from build123d import *

# Parameters (mm, degrees)
BOSS_EXTRUDE1_DEPTH = 1.5875
SKETCH2_W           = 43
SKETCH2_H           = 127
BOSS_EXTRUDE2_DEPTH = 1.5875


with BuildPart() as part:
    # Sketch1 → Boss-Extrude1 (new body)
    with BuildSketch(Plane.XY):
        Polygon((-117, 99.5), (-103.5, 116.5), (-103.5, 120), (-146.5, 120), (-146.5, 116.5), (-133, 99.5), (-133, 20.5), (-146.5, 3.5), (-146.5, 0), (-103.5, 0), (-103.5, 3.5), (-117, 20.5), align=None)
        with BuildLine():
            ThreePointArc((-134.15, 112.5), (-132.5, 110.85), (-130.85, 112.5))
            ThreePointArc((-130.85, 112.5), (-132.5, 114.15), (-134.15, 112.5))
        make_face(mode=Mode.SUBTRACT)
        with BuildLine():
            ThreePointArc((-119.15, 112.5), (-117.5, 110.85), (-115.85, 112.5))
            ThreePointArc((-115.85, 112.5), (-117.5, 114.15), (-119.15, 112.5))
        make_face(mode=Mode.SUBTRACT)
        with BuildLine():
            ThreePointArc((-115.85, 7.5), (-117.5, 9.15), (-119.15, 7.5))
            ThreePointArc((-119.15, 7.5), (-117.5, 5.85), (-115.85, 7.5))
        make_face(mode=Mode.SUBTRACT)
        with BuildLine():
            ThreePointArc((-134.15, 7.5), (-132.5, 5.85), (-130.85, 7.5))
            ThreePointArc((-130.85, 7.5), (-132.5, 9.15), (-134.15, 7.5))
        make_face(mode=Mode.SUBTRACT)
    extrude(amount=BOSS_EXTRUDE1_DEPTH)

    # Sketch2 → Boss-Extrude2 (add)
    with BuildSketch(Plane(origin=(0, 120, 0), x_dir=(1, 0, 0), z_dir=(0, 1, 0))):
        with Locations((-125, 61.9125)):
            Rectangle(SKETCH2_W, SKETCH2_H)
    extrude(amount=BOSS_EXTRUDE2_DEPTH)


solid = part.part
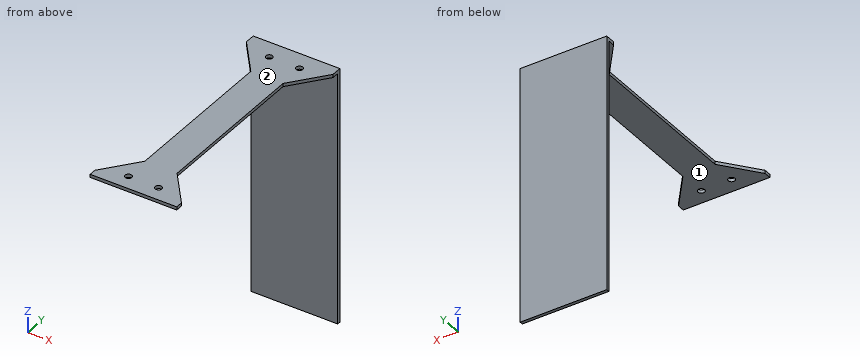
Input: part model. Units: mm. Frame: model coordinates. Face numbers are marked on the shaded views. A direction names the side the tool comes from. Coordinates: 2 decimals unless noted, no trailing zeros. Loops run counter-clockwise (first coordinate to the right, second up) from the corner with the lowest first, then second, coordinate; pieces in that order, holes last.
(1) Set-up query: the marked faces 1 and 2. Return all of +Z, -Z, +X, -X, +Y, -Y with unobstructed straight access to the full face (end or side cutting, diameter ignored); none if empty.
(2) Section C-C on x = -123. Return the cut outline in (y, z).
(3) Section A-A on y = 112.5. Return the cut outline in (x, z), then the cut area to 3 significant figures.
(4) Section B-B on x = -113. Return the cut outline in (y, z), then the cut area to 3 significant figures.
(5) Material intervals for probe 1 along Y at (x, z) = (-132.5, 0.45); probe 2 along Y at (x, z) = (-116, -56.5); probe 3 along Z at (x, y) = (-128, 23), sorted ascending.
(6) First-contact query: pin 1 Ø1.7 at (y, z) = (52.5, 0.5) entering from -X; pin 2 Ø4 at (x, y) = (-133.5, 98.5) entering from -Z; pin 3 Ø13 at (x, z) = (-117.5, -34.5) entering from -Y. Flat tips, straight axial feed; report the tip coordinate or a pass-through.
(7) Section D-D on y = 81. Return the cut outline in (x, z), then the cut area to 3 significant figures.
Data:
1. face 1: -Z, +X, -X, -Y
1. face 2: +Z, +X, -X, +Y, -Y
2. outline: (0, 0) - (120, 0) - (120, -125.41) - (121.59, -125.41) - (121.59, 1.59) - (0, 1.59) - close
3. outline: (-143.32, 0) - (-134.15, 0) - (-134.15, 1.59) - (-143.32, 1.59) - close; (-130.85, 0) - (-119.15, 0) - (-119.15, 1.59) - (-130.85, 1.59) - close; (-115.85, 0) - (-106.68, 0) - (-106.68, 1.59) - (-115.85, 1.59) - close
3. area: 47.7 mm2
4. outline: (0, 0) - (15.46, 0) - (15.46, 1.59) - (0, 1.59) - close; (104.54, 0) - (120, 0) - (120, -125.41) - (121.59, -125.41) - (121.59, 1.59) - (104.54, 1.59) - close
4. area: 251 mm2
5. probe 1: y = 0 to 5.85, 9.15 to 110.85, 114.15 to 121.59
5. probe 2: y = 120 to 121.59
5. probe 3: z = 0 to 1.59
6. pin 1: stops at x = -133
6. pin 2: stops at z = 0
6. pin 3: stops at y = 120
7. outline: (-133, 0) - (-117, 0) - (-117, 1.59) - (-133, 1.59) - close
7. area: 25.4 mm2
